```python
from build123d import *

# Parameters (mm, degrees)
F0_R     = 30
F0_R_2   = 3
F1_DEPTH = 25
F2_START = 2
F0_R_3   = 2.75
F2_DEPTH = 21
F4_DEPTH = 6
F5_START = 19
F5_DEPTH = 4


# Not quite as in the source:
# - a fillet or chamfer that OpenCascade refuses, or shapes differently, is made with other operations: its cross-section is extruded or revolved along the edge and cut away or added
# - a feature names something its author has since deleted; it is built from what else it names


with BuildPart() as f1:
    # F0 (on Top) → F1 (new body)
    with BuildSketch(Plane.XY):
        Circle(F0_R)
        with BuildLine():
            ThreePointArc((16.2480768093, 5), (16.8109682314, 2.5281113744), (17, 0))
            ThreePointArc((17, 0), (16.8109682314, -2.5281113744), (16.2480768093, -5))
            ThreePointArc((16.2480768093, -5), (12.0208152802, -12.0208152802), (5, -16.2480768093))
            ThreePointArc((5, -16.2480768093), (0, -17), (-5, -16.2480768093))
            ThreePointArc((-5, -16.2480768093), (-12.0208152802, -12.0208152802), (-16.2480768093, -5))
            ThreePointArc((-16.2480768093, -5), (-17, 0), (-16.2480768093, 5))
            ThreePointArc((-16.2480768093, 5), (-12.0208152802, 12.0208152802), (-5, 16.2480768093))
            ThreePointArc((-5, 16.2480768093), (0, 17), (5, 16.2480768093))
            ThreePointArc((5, 16.2480768093), (12.0208152802, 12.0208152802), (16.2480768093, 5))
        make_face(mode=Mode.SUBTRACT)
        with BuildLine():
            ThreePointArc((16.2480768093, -5), (16.8109682314, -2.5281113744), (17, 0))
            ThreePointArc((17, 0), (16.8109682314, 2.5281113744), (16.2480768093, 5))
            ThreePointArc((16.2480768093, 5), (10.4163777832, 1.9103772572), (4.2426406998, 4.2426406745))
            ThreePointArc((4.2426406998, 4.2426406745), (5.5432771985, 2.2961005859), (6, 0))
            ThreePointArc((6, 0), (5.5432771928, -2.2961005997), (4.2426406787, -4.2426406956))
            ThreePointArc((4.2426406787, -4.2426406956), (10.4163777683, -1.9103772563), (16.2480768093, -5))
        make_face()
        with BuildLine():
            ThreePointArc((4.2426406998, 4.2426406745), (1.9103772561, 10.4163777654), (5, 16.2480768093))
            ThreePointArc((5, 16.2480768093), (0, 17), (-5, 16.2480768093))
            ThreePointArc((-5, 16.2480768093), (-1.9103772567, 10.4163777743), (-4.2426406871, 4.2426406871))
            ThreePointArc((-4.2426406871, 4.2426406871), (8.9e-09, 6), (4.2426406998, 4.2426406745))
        make_face()
        with BuildLine():
            ThreePointArc((6, 0), (5.5432771985, 2.2961005859), (4.2426406998, 4.2426406745))
            ThreePointArc((4.2426406998, 4.2426406745), (8.9e-09, 6), (-4.2426406871, 4.2426406871))
            ThreePointArc((-4.2426406871, 4.2426406871), (-6, 4e-10), (-4.2426406877, -4.2426406865))
            ThreePointArc((-4.2426406877, -4.2426406865), (-6.4e-09, -6), (4.2426406787, -4.2426406956))
            ThreePointArc((4.2426406787, -4.2426406956), (5.5432771928, -2.2961005997), (6, 0))
        make_face()
        Polygon((0, -4.5033320997), (-3.9, -2.2516660498), (-3.9, 2.2516660498), (0, 4.5033320997), (3.9, 2.2516660498), (3.9, -2.2516660498), align=None, mode=Mode.SUBTRACT)
        with BuildLine():
            ThreePointArc((-5, -16.2480768093), (0, -17), (5, -16.2480768093))
            ThreePointArc((5, -16.2480768093), (1.910377257, -10.4163777803), (4.2426406787, -4.2426406956))
            ThreePointArc((4.2426406787, -4.2426406956), (-6.4e-09, -6), (-4.2426406877, -4.2426406865))
            ThreePointArc((-4.2426406877, -4.2426406865), (-1.9103772566, -10.4163777739), (-5, -16.2480768093))
        make_face()
        with BuildLine():
            ThreePointArc((-4.2426406877, -4.2426406865), (-6, 4e-10), (-4.2426406871, 4.2426406871))
            ThreePointArc((-4.2426406871, 4.2426406871), (-10.4163777743, 1.9103772567), (-16.2480768093, 5))
            ThreePointArc((-16.2480768093, 5), (-17, 0), (-16.2480768093, -5))
            ThreePointArc((-16.2480768093, -5), (-10.4163777747, -1.9103772567), (-4.2426406877, -4.2426406865))
        make_face()
        Polygon((-3.9, 2.2516660498), (-3.9, -2.2516660498), (0, -4.5033320997), (3.9, -2.2516660498), (3.9, 2.2516660498), (0, 4.5033320997), align=None)
        Circle(F0_R_2, mode=Mode.SUBTRACT)
    extrude(amount=F1_DEPTH)

    # F0 (on Top) → F2 (join)
    with BuildSketch(Plane.XY.offset(F2_START)):
        Circle(F0_R_2)
        Circle(F0_R_3, mode=Mode.SUBTRACT)
    extrude(amount=F2_DEPTH)

    # F3: chamfer of 5 on 2 edges, made by hand


with BuildPart() as f3_tool2:
    # F3_s3 → F3_t4 (revolve)
    with BuildSketch(Plane.XZ):
        Polygon((8, 0), (3, 5), (3, 0), align=None)
    revolve(axis=Axis((0, 0, 0), (0, 0, 1)))

    split(bisect_by=Plane.XY.offset(2), keep=Keep.BOTTOM)


with BuildPart() as f1_1:
    add(f1.part)

    # F3_t1: cut F3_tool2
    add(f3_tool2.part, mode=Mode.SUBTRACT)


with BuildPart() as f3_tool7:
    # F3_s8 → F3_t9 (revolve)
    with BuildSketch(Plane.XZ):
        Polygon((8, 25), (3, 20), (3, 25), align=None)
    revolve(axis=Axis((0, 0, 25), (0, 0, 1)))

    split(bisect_by=Plane.XY.offset(23), keep=Keep.TOP)


with BuildPart() as f1_2:
    add(f1_1.part)

    # F3_t6: cut F3_tool7
    add(f3_tool7.part, mode=Mode.SUBTRACT)

    # F0 (on Top) → F4 (cut)
    with BuildSketch(Plane.XY):
        Polygon((-3.9, 2.2516660498), (-3.9, -2.2516660498), (0, -4.5033320997), (3.9, -2.2516660498), (3.9, 2.2516660498), (0, 4.5033320997), align=None)
        Circle(F0_R_2, mode=Mode.SUBTRACT)
        Circle(F0_R_2)
        Circle(F0_R_3, mode=Mode.SUBTRACT)
        Circle(F0_R_3)
    extrude(amount=F4_DEPTH, mode=Mode.SUBTRACT)

    # F0 (on Top) → F5 (cut)
    with BuildSketch(Plane.XY.offset(F5_START)):
        Polygon((-3.9, 2.2516660498), (-3.9, -2.2516660498), (0, -4.5033320997), (3.9, -2.2516660498), (3.9, 2.2516660498), (0, 4.5033320997), align=None)
        Circle(F0_R_2, mode=Mode.SUBTRACT)
        Circle(F0_R_2)
        Circle(F0_R_3, mode=Mode.SUBTRACT)
    extrude(amount=F5_DEPTH, mode=Mode.SUBTRACT)


solid = f1_2.part
```
Geometry: final body of the model. Coordinates: model frame, mm. A direction names the side the tool comes from. Round coordinates to 2 decimals unless told otherwise and drop trailing zeros. Order: outer loops, then holes, each group sorted by start corner. A loop starts at its lowest first (then second) coordinate and runs counter-clockwise, first axis right, second up. Notation, with made-up numbers: M -36,19.5 L 3,19.5 A3 cw 3,23.5 Z; hole C 31.25,54 d10. An arc over 180 degrees is marked long. One line per item, written item: value.
(1) Pull-direction query (Y, two-part tool) for faces 4 (the cylindrical face through (-29.97, 1.32, 12.32)), 5 (the flat face through (-1.98, -3.36, 20.97)); classes: pulls with the +Y half, pulls with the -Y half, needs draft (parallel to the pull), parting line crosses it, or undercut.
Result sheet:
face 4: parting line crosses it
face 5: undercut
(2) Cut plane A-A (z = 21). Return the cut outline in (x, y).
Result sheet:
outline: C 0,0 d60; hole M -16.25,-5 A17 ccw -5,-16.25 A8.02 ccw long Z; hole M -16.25,5 A8.02 ccw long -5,16.25 A17 ccw Z; hole M -3.9,-2.25 L 0,-4.5 L 3.9,-2.25 L 3.9,2.25 L 0,4.5 L -3.9,2.25 Z; hole M 5,-16.25 A17 ccw 16.25,-5 A8.02 ccw long Z; hole M 5,16.25 A8.02 ccw long 16.25,5 A17 ccw Z
(3) Reachability of faces 1 (the cylindrical face through (-12.1, 11.94, 12.32)), 2 (the flat face through (3.9, 0, 21)), 3 (the conical face through (-7, 0, 1)) from +Z, -Z, +X, -X, +Y, -Y: full face, straight path, thin tool, end or side. Return the list, or none.
Result sheet:
face 1: +Z, -Z
face 2: +Z
face 3: -Z
(4) Line query: probe 1 along Y at (x, z) = (0, 16); probe 2 along Y at (x, z) = (11, 11.25); probe 3 along Y at (x, z) = (-13, 10.25). Output: solid intervals per line, ascending. Write a range as [from, to].
Result sheet:
probe 1: [-30, -2.75], [2.75, 30]
probe 2: [-27.91, -12.96], [-1.97, 1.97], [12.96, 27.91]
probe 3: [-27.04, -10.95], [-2.51, 2.51], [10.95, 27.04]
(5) Pin query (flat end, axial travel): P1, Ø7, axis at x = 0, y = 0, coming from the +Z side; P2, Ø8.5, axis at x = -0.5, y = 0, coming from the -Z side; P3, Ø2, axis at x = -11, z = 3.5, coming from the -Y side. Return the tip coordinate at first contact, or that it passes through.
Result sheet:
P1: z = 19
P2: z = 2
P3: y = -28.28
(6) Cut plane C-C (x = 13). Return the cut outline in (y, z), and give its area (3 significant figures).
Result sheet:
outline: M -27.04,0 L -10.95,0 L -10.95,25 L -27.04,25 Z; M -2.51,0 L 2.51,0 L 2.51,25 L -2.51,25 Z; M 10.95,0 L 27.04,0 L 27.04,25 L 10.95,25 Z
area: 930 mm2
(7) Cut plane B-B (y = 0). Return the cut outline in (x, z).
Result sheet:
outline: M -30,0 L -8,0 L -6,2 L -3.9,2 L -3.9,6 L -2.75,6 L -2.75,19 L -3.9,19 L -3.9,23 L -6,23 L -8,25 L -30,25 Z; M 2.75,6 L 3.9,6 L 3.9,2 L 6,2 L 8,0 L 30,0 L 30,25 L 8,25 L 6,23 L 3.9,23 L 3.9,19 L 2.75,19 Z
(8) Cut plane D-D (y = -14.5). Return the cut outline in (x, z), and give its area (3 significant figures).
Result sheet:
outline: M -26.26,0 L -8.87,0 L -8.87,25 L -26.26,25 Z; M -3.34,0 L 3.34,0 L 3.34,25 L -3.34,25 Z; M 8.87,0 L 26.26,0 L 26.26,25 L 8.87,25 Z
area: 1,040 mm2
